Can you work these out from the model? Positions are in its coordinate system, mm. Round coordinates to 2 decimals unless told otherwise and drop trailing zeros. Loops run counter-clockwise (first coordinate to the right, second up) from the corner with the lowest first, then second, coordinate; pieces in that order, holes last.
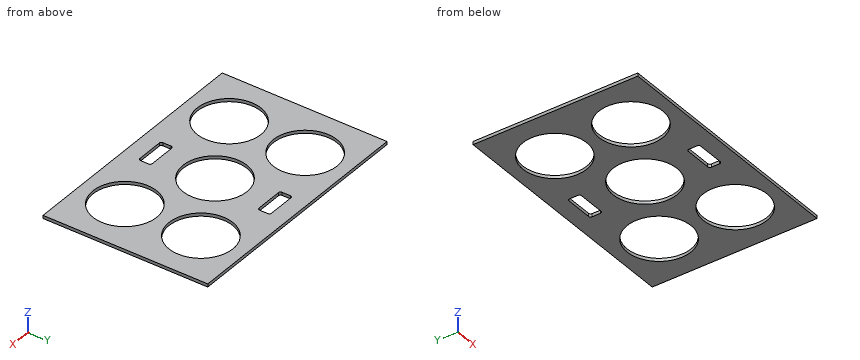
from build123d import *

# Parameters (mm, degrees)
F0_W     = 1195
F0_H     = 795
F0_R     = 154
F1_DEPTH = 15


with BuildPart() as f1:
    # F0 (on Top) → F1 (new body)
    with BuildSketch(Plane.XY):
        with Locations((444.978323, 111.086236)):
            Rectangle(F0_W, F0_H)
        with BuildLine():
            ThreePointArc((367.478323, -156.413764), (370.407255, -149.342696), (377.478323, -146.413764))
            Line((377.478323, -146.413764), (507.478323, -146.413764))
            ThreePointArc((507.478323, -146.413764), (514.549391, -149.342696), (517.478323, -156.413764))
            Line((517.478323, -156.413764), (517.478323, -196.413764))
            ThreePointArc((517.478323, -196.413764), (514.549391, -203.484832), (507.478323, -206.413764))
            Line((507.478323, -206.413764), (377.478323, -206.413764))
            ThreePointArc((377.478323, -206.413764), (370.407255, -203.484832), (367.478323, -196.413764))
            Line((367.478323, -196.413764), (367.478323, -156.413764))
        make_face(mode=Mode.SUBTRACT)
        with Locations((97.478323, -72.413764)):
            Circle(F0_R, mode=Mode.SUBTRACT)
        with Locations((444.978323, 111.086236)):
            Circle(F0_R, mode=Mode.SUBTRACT)
        with Locations((792.478323, -72.413764)):
            Circle(F0_R, mode=Mode.SUBTRACT)
        with Locations((97.478323, 294.586236)):
            Circle(F0_R, mode=Mode.SUBTRACT)
        with BuildLine():
            ThreePointArc((367.478323, 418.586236), (370.407255, 425.657304), (377.478323, 428.586236))
            Line((377.478323, 428.586236), (507.478323, 428.586236))
            ThreePointArc((507.478323, 428.586236), (514.549391, 425.657304), (517.478323, 418.586236))
            Line((517.478323, 418.586236), (517.478323, 378.586236))
            ThreePointArc((517.478323, 378.586236), (514.549391, 371.515168), (507.478323, 368.586236))
            Line((507.478323, 368.586236), (377.478323, 368.586236))
            ThreePointArc((377.478323, 368.586236), (370.407255, 371.515168), (367.478323, 378.586236))
            Line((367.478323, 378.586236), (367.478323, 418.586236))
        make_face(mode=Mode.SUBTRACT)
        with Locations((792.478323, 294.586236)):
            Circle(F0_R, mode=Mode.SUBTRACT)
    extrude(amount=F1_DEPTH)


solid = f1.part
(1) If I drill on line 1 (Y direction, x = 442, z = 10.5); line 2 (X direction, y = -76, z = 4); line 3 (Y direction, x = 87, z = 3.75), over which ranges is the centre line in solid material (lowest first)?
Worked answers:
line 1: y = -286.41 to -206.41, -146.41 to -42.88, 265.06 to 368.59, 428.59 to 508.59
line 2: x = -152.52 to -56.48, 251.44 to 638.52, 946.44 to 1042.48
line 3: y = -286.41 to -226.06, 81.23 to 140.94, 448.23 to 508.59
(2) If we section it at D-D, the plane y = 328: List the corners of the cut face in (x, z) for me.
Worked answers:
outline: (-152.52, 0) - (-52.85, 0) - (-52.85, 15) - (-152.52, 15) - close; (247.81, 0) - (642.15, 0) - (642.15, 15) - (247.81, 15) - close; (942.81, 0) - (1042.48, 0) - (1042.48, 15) - (942.81, 15) - close
(3) If we section it at C-C, the plane x = 539.5: List the corners of the cut face in (y, z) for me.
Worked answers:
outline: (-286.41, 0) - (-10.49, 0) - (-10.49, 15) - (-286.41, 15) - close; (232.67, 0) - (508.59, 0) - (508.59, 15) - (232.67, 15) - close
(4) If we section it at B-B, the plane y = 229: List the corners of the cut face in (x, z) for me.
Worked answers:
outline: (-152.52, 0) - (-41.86, 0) - (-41.86, 15) - (-152.52, 15) - close; (236.81, 0) - (345.92, 0) - (345.92, 15) - (236.81, 15) - close; (544.04, 0) - (653.14, 0) - (653.14, 15) - (544.04, 15) - close; (931.81, 0) - (1042.48, 0) - (1042.48, 15) - (931.81, 15) - close
(5) If we section it at A-A, the plane x = 676: List the corners of the cut face in (y, z) for me.
Worked answers:
outline: (-286.41, 0) - (-173.16, 0) - (-173.16, 15) - (-286.41, 15) - close; (28.33, 0) - (193.84, 0) - (193.84, 15) - (28.33, 15) - close; (395.33, 0) - (508.59, 0) - (508.59, 15) - (395.33, 15) - close
